from build123d import *

# Parameters (mm, degrees)
SKETCH1_R           = 4.75
BOSS_EXTRUDE1_DEPTH = 2.5


with BuildPart() as part:
    # Sketch1 → Boss-Extrude1 (new, symmetric)
    with BuildSketch(Plane.YZ):
        with BuildLine():
            Line((-15.757717512, 0), (-5, 0))
            Line((-5, 0), (-5, -5))
            Line((-5, -5), (5, -5))
            Line((5, -5), (5, 0))
            Line((5, 0), (14.242282488, 0))
            Line((14.242282488, 0), (12.716235334, 20.927285791))
            ThreePointArc((12.716235334, 20.927285791), (0.446501859, 32.742179409), (-12.620138577, 21.815103933))
            Line((-12.620138577, 21.815103933), (-15.757717512, 0))
        make_face()
        with Locations(Location((0, 20, 0), (0, 0, 270))):
            Circle(SKETCH1_R, mode=Mode.SUBTRACT)
    extrude(amount=BOSS_EXTRUDE1_DEPTH, both=True)


solid = part.part
CAD build for the part. Positions are in the model's coordinates, mm. A direction names the side the tool comes from. Coordinates: 2 decimals unless noted, no trailing zeros. Write each loop counter-clockwise with the first axis right and the second up, starting at its lowest first coordinate (ties: lowest second). Pieces come first, ordered by that corner, then holes. Notation, with made-up numbers: M 52,-20.75 L 81,-20.75 A20 ccw 81,16.25 Z; hole C 48,-13 d11. An arc over 180 degrees is marked long. Return JSON: item names as keys, results as strings.
Item 1: Slice it at B-B, the plane x = 1.4. Write the cut outline in (y, z).
Findings below:
{"outline": "M -15.76,0 L -5,0 L -5,-5 L 5,-5 L 5,0 L 14.24,0 L 12.72,20.93 A12.75 ccw -12.62,21.82 Z; hole C 0,20 d9.5"}
Item 2: Slice it at D-D, the plane z = -1.5. Write the cut outline in (x, y), and give its area (3 significant figures).
Findings below:
{"outline": "M -2.5,-5 L 2.5,-5 L 2.5,5 L -2.5,5 Z", "area": "50.0 mm2"}
Item 3: Two-plate mould, pull along Y, no slides. Class faces 1 (the flat face through (0, -10, 0)), 2 (the flat face through (0, 5, -3)), 3 (the cylindrical face through (-0.035, -1.819, 15.612)): +Y half, -Y half, draft (parallel to the pull), parting line (faces both ways), or undercut.
Findings below:
{"face 1": "draft", "face 2": "+Y half", "face 3": "undercut"}
Item 4: Slice it at C-C, the plane z = 20. Write the cut outline in (x, y).
Findings below:
{"outline": "M -2.5,-12.88 L 2.5,-12.88 L 2.5,-4.75 L -2.5,-4.75 Z; M -2.5,4.75 L 2.5,4.75 L 2.5,12.78 L -2.5,12.78 Z"}
Item 5: Slice it at A-A, the plane y = 0. Write the cut outline in (x, z), and give its area (3 significant figures).
Findings below:
{"outline": "M -2.5,-5 L 2.5,-5 L 2.5,15.25 L -2.5,15.25 Z; M -2.5,24.75 L 2.5,24.75 L 2.5,32.75 L -2.5,32.75 Z", "area": "141 mm2"}
Item 6: Probe line 1 (Y direction, x = 1.1, z = 21.5); line 2 (Y direction, x = 1.4, z = -3); line 3 (Z direction, x = 0, y = -3.75). List the from-to ranges inside material, lowest first. Write a range as from..to.
Findings below:
{"line 1": "y = -12.67..-4.51, 4.51..12.66", "line 2": "y = -5..5", "line 3": "z = -5..17.08, 22.92..32.19"}
Item 7: Drop flat-ended pins along their axis: pin 1 Ø12.5 at (y, z) = (0, 20) entering from -X; pin 2 Ø1.5 at (x, y) = (0, 6.5) entering from +Z; pin 3 Ø1.5 at (x, y) = (1, -10) entering from -Z; pin 4 Ø3 at (x, z) = (0.5, 13.5) entering from +Y. Give the stop position or say it passes through.
Findings below:
{"pin 1": "stops at x = -2.5", "pin 2": "stops at z = 31.38", "pin 3": "stops at z = 0", "pin 4": "stops at y = 13.37"}
Item 8: Which spindle directions (+Z, -Z, +X, -X, +Y, -Y) get a long thin tool onto all of the face, cutting with end or side? Do faces 4 (the flat face through (0, -5, -2)), 5 (the flat face through (0, 10, 0)), 6 (the flat face through (-2.5, -1, 14)). Say none if no direction does.
Findings below:
{"face 4": "-Z, +X, -X, -Y", "face 5": "-Z, +X, -X, +Y", "face 6": "+Z, -Z, -X, +Y, -Y"}
